Design review of the part built by this model. Coordinates are the model's own, in mm. A direction names the side the tool comes from. Give positions to 0.01 mm unless a question says otherwise; leave off trailing zeros. Order: outer loops, then holes, each group sorted by start corner. A loop starts at its lowest first (then second) coordinate and runs counter-clockwise, first axis right, second up.
```python
from build123d import *

# Parameters (mm, degrees)
F1_DEPTH  = 30
F2_R      = 1
F2_R_2    = 0.0533765033
F3_DEPTH  = 30.001
F4_R      = 10
F5_DEPTH  = 64
F8_DEPTH  = 30
F9_W      = 5.2633735355
F9_H      = 23.3362393919
F10_DEPTH = 25
F11_W     = 8.7402192639
F11_H     = 1.3938806951
F12_DEPTH = 30
F13_DEPTH = 41.9052980466


with BuildPart() as f1:
    # F0 (on Top) → F1 (new body)
    with BuildSketch(Plane.XY):
        with BuildLine():
            Line((-101.3173758984, 35), (-101.3173758984, 0))
            Line((-101.3173758984, 0), (101.8826241016, 0))
            ThreePointArc((101.8826241016, 0), (56.0897429361, 9.5394690074), (9.8705293288, 16.7348653069))
            ThreePointArc((9.8705293288, 16.7348653069), (4.9096577711, 18.5604467569), (0, 20.5195932071))
            ThreePointArc((0, 20.5195932071), (-49.491894157, 35.9236891605), (-101.3173758984, 35))
        make_face()
    extrude(amount=F1_DEPTH)

    # F2 (on Top) → F3 (cut, through all)
    with BuildSketch(Plane.XY):
        with Locations((-87.232263687, 3)):
            Circle(F2_R)
        with Locations((60.264059, 3)):
            Circle(F2_R_2)
        with Locations((-2.4870128836, 3)):
            Circle(F2_R)
    extrude(amount=F3_DEPTH, mode=Mode.SUBTRACT)

    # F4 (on face) → F5 (cut)
    with BuildSketch(Plane(origin=(-101.3173758984, 0, 0), x_dir=(0, -1, 0), z_dir=(-1, 0, 0))):
        with Locations((-16.8194788357, 14.8095988691)):
            Circle(F4_R)
    extrude(amount=-F5_DEPTH, mode=Mode.SUBTRACT)

    # F7 (on face) → F8 (join)
    with BuildSketch(Plane.XY.offset(30)):
        with BuildLine():
            Line((-100.0109697279, 40.5104173515), (-99.8982514965, 35.248250918))
            add(Edge.make_bspline(
                [(-99.8982514965, 35.248250918), (-99.1698783521, 35.2086363528), (-95.596989963, 35.7161657204), (-94.9947075015, 36.0070484152)],
                knots=[0, 0, 0, 0, 4.9619066248, 4.9619066248, 4.9619066248, 4.9619066248], degree=3))
            Line((-94.9947075015, 36.0070484152), (-94.9947075015, 40.5104173515))
            Line((-94.9947075015, 40.5104173515), (-100.0109697279, 40.5104173515))
        make_face()
    extrude(amount=-F8_DEPTH)

    # F9 (on face) → F10 (cut)
    with BuildSketch(Plane(origin=(-99.0977465794, -2.122723191, 0), x_dir=(0.0214155865, -0.99977066, 0), z_dir=(-0.99977066, -0.0214155865, 0))):
        with Locations((-40.0112335009, 14.7758348612)):
            Rectangle(F9_W, F9_H)
    extrude(amount=-F10_DEPTH, mode=Mode.SUBTRACT)

    # F11 (on face) → F12 (join)
    with BuildSketch(Plane.XY.offset(30)):
        with Locations((-97.0257730341, 41.2073576991)):
            Rectangle(F11_W, F11_H)
    extrude(amount=-F12_DEPTH)

    # F6 (on face) → F13 (cut, through all)
    with BuildSketch(Plane.XZ):
        Polygon((0, 30), (101.8826241016, 15), (101.8826241016, 30), align=None)
        Polygon((101.8826241016, 15), (0, 0), (101.8826241016, 0), align=None)
    extrude(amount=-F13_DEPTH, mode=Mode.SUBTRACT)


solid = f1.part
```
1. Take a section at B-B (x = -67). State the section outline as (y, z) points.
Recorded:
outline: (0, 0) - (37.47, 0) - (37.47, 30) - (0, 30) - close; hole circle Ø20 at (16.82, 14.81)
2. Take a section at D-D (y = 24.5). State the section outline as (x, z) points, then the cut area to 3 significant figures.
Recorded:
outline: (-101.32, 0) - (-8.63, 0) - (-8.63, 30) - (-101.32, 30) - (-101.32, 21.21) - (-37.32, 21.21) - (-37.32, 8.41) - (-101.32, 8.41) - close
area: 1,960 mm2
3. For line 1 along Y through (x, z) = (10, 1.75); line 2 along Y through (x, z) = (-91.5, 16); line 3 along Y through (x, z) = (-76, 25), list the stretches that pass through material, from the lowest coordinate up.
Recorded:
line 1: y = 0 to 16.72
line 2: y = 0 to 6.89, 26.75 to 35.43
line 3: y = 0 to 35.76
4. For pin 1 (4 mm diameter, centred on x = -76.5, z = 22.5, fed in from +Y); pin 2 (1.5 mm diameter, centred on x = -13.5, y = 14, fed in from -Z); pin 3 (2 mm diameter, centred on x = -40, z = 18.5, fed in from +Y); pin 4 (9 mm diameter, centred on y = 19.5, z = 12.5, fed in from -X), all flat-tipped, find the tip position at first contact; note any pin that passes through.
Recorded:
pin 1: stops at y = 37.55
pin 2: stops at z = 0
pin 3: stops at y = 34.48
pin 4: stops at x = -37.32
5. Draft analysis for pull direction Z (two halves, no side actions). For faces 1 (the face through (-51, 17, 30)), 2 (the face through (-97, 40.51, 15)), 3 (the face through (-97, 41.904, 15)), state which applies: pulls with the +Z half, pulls with the -Z half, needs draft (parallel to the pull), parting line crosses it, or undercut.
Recorded:
face 1: pulls with the +Z half
face 2: undercut
face 3: needs draft
6. Machinability: for faces 4 (the face through (-69.77, 7.28, 17.81)), 5 (the face through (-94.995, 38, 28)), which of the approach directions +Z, -Z, +X, -X, +Y, -Y give a long, thin tool a straight path to every point of the face, cutting with its end or side? Answer none if there is none.
Recorded:
face 4: -X
face 5: +Z, -Z
7. Take a section at C-C (x = -33.5). State the section outline as (y, z) points.
Recorded:
outline: (0, 0) - (32.82, 0) - (32.82, 30) - (0, 30) - close
